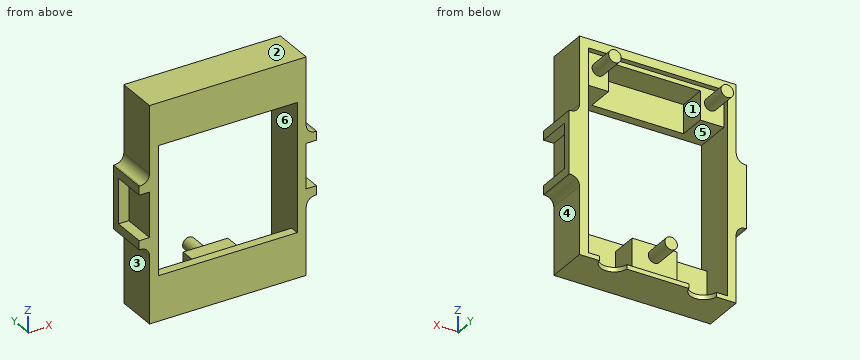
```python
from build123d import *

# Parameters (mm, degrees)
SKETCH1_W           = 35
SKETCH1_H           = 48
BOSS_EXTRUDE1_DEPTH = 2
SKETCH2_W           = 35
SKETCH2_H           = 48
SKETCH2_W_2         = 31
SKETCH2_H_2         = 44
BOSS_EXTRUDE2_DEPTH = 7.3
SKETCH3_W           = 10
SKETCH3_H           = 7
SKETCH3_W_2         = 5.25
SKETCH3_H_2         = 6.4
BOSS_EXTRUDE3_DEPTH = 6.1
CUT_EXTRUDE5_DEPTH  = 1
SKETCH10_W          = 31
SKETCH10_H          = 28.6
CUT_EXTRUDE6_DEPTH  = 31.586598372
BOSS_EXTRUDE4_START = 8.1
SKETCH8_R           = 1.4
BOSS_EXTRUDE4_DEPTH = 6
SKETCH14_W          = 2.3
SKETCH14_H          = 1.8
BOSS_EXTRUDE6_DEPTH = 5
SKETCH15_W          = 2
SKETCH15_H          = 9.3
BOSS_EXTRUDE7_DEPTH = 2.3
FILLET3_R           = 2
SKETCH16_W          = 31
SKETCH16_H          = 1
CUT_EXTRUDE8_DEPTH  = 1.2


with BuildPart() as part:
    # Sketch1 → Boss-Extrude1 (new body)
    with BuildSketch(Plane(origin=(0, 0, 0), x_dir=(1, 0, 0), z_dir=(0, 1, 0))):
        Rectangle(SKETCH1_W, SKETCH1_H)
    extrude(amount=BOSS_EXTRUDE1_DEPTH)

    # Sketch2 → Boss-Extrude2 (add)
    with BuildSketch(Plane(origin=(0, 2, 0), x_dir=(1, 0, 0), z_dir=(0, 1, 0))):
        Rectangle(SKETCH2_W, SKETCH2_H)
        with Locations((0, 1)):
            Rectangle(SKETCH2_W_2, SKETCH2_H_2, mode=Mode.SUBTRACT)
    extrude(amount=BOSS_EXTRUDE2_DEPTH)

    # Sketch3 → Boss-Extrude3 (add)
    with BuildSketch(Plane(origin=(0, 2, 0), x_dir=(1, 0, 0), z_dir=(0, 1, 0))):
        with Locations((0, 19.5)):
            Rectangle(SKETCH3_W, SKETCH3_H)
        with Locations((-12.875, -17.8)):
            Rectangle(SKETCH3_W_2, SKETCH3_H_2)
        with Locations((12.875, -17.8)):
            Rectangle(SKETCH3_W_2, SKETCH3_H_2)
    extrude(amount=BOSS_EXTRUDE3_DEPTH)

    # Sketch6 → Cut-Extrude5 (cut)
    with BuildSketch(Plane(origin=(0, 0, -24), x_dir=(-1, 0, 0), z_dir=(0, 0, -1))):
        with BuildLine():
            ThreePointArc((-13.059411708, 9.3), (-10, 6.7), (-6.940588292, 9.3))
            Line((-6.940588292, 9.3), (-13.059411708, 9.3))
        make_face()
        with BuildLine():
            Line((13.059411708, 9.3), (6.940588292, 9.3))
            ThreePointArc((6.940588292, 9.3), (10, 6.7), (13.059411708, 9.3))
        make_face()
    extrude(amount=-CUT_EXTRUDE5_DEPTH, mode=Mode.SUBTRACT)

    # Sketch10 → Cut-Extrude6 (cut, through all)
    with BuildSketch(Plane(origin=(0, 2, 0), x_dir=(1, 0, 0), z_dir=(0, 1, 0))):
        with Locations((0, -0.3)):
            Rectangle(SKETCH10_W, SKETCH10_H)
    extrude(amount=-CUT_EXTRUDE6_DEPTH, mode=Mode.SUBTRACT)

    # Sketch8 → Boss-Extrude4 (add)
    with BuildSketch(Plane(origin=(0, 0, 0), x_dir=(1, 0, 0), z_dir=(0, 1, 0)).offset(BOSS_EXTRUDE4_START)):
        with Locations(Location((-12.55, -18.7, 0), (0, 0, 90))):
            Circle(SKETCH8_R)
        with Locations(Location((12.55, -18.7, 0), (0, 0, 270))):
            Circle(SKETCH8_R)
        with Locations(Location((0, 18.6, 0), (0, 0, 270))):
            Circle(SKETCH8_R)
    extrude(amount=BOSS_EXTRUDE4_DEPTH)

    # Sketch14 → Boss-Extrude6 (add, symmetric)
    with BuildSketch(Plane.XY):
        with Locations((18.65, 8.4)):
            Rectangle(SKETCH14_W, SKETCH14_H)
    boss_extrude6 = extrude(amount=BOSS_EXTRUDE6_DEPTH, both=True)

    # Sketch15 → Boss-Extrude7 (add)
    with BuildSketch(Plane(origin=(17.5, 0, 0), x_dir=(0, 0, -1), z_dir=(1, 0, 0))):
        with Locations((-6, 4.65)):
            Rectangle(SKETCH15_W, SKETCH15_H)
        with Locations((6, 4.65)):
            Rectangle(SKETCH15_W, SKETCH15_H)
    boss_extrude7 = extrude(amount=BOSS_EXTRUDE7_DEPTH)

    # Mirror3: Boss-Extrude6, Boss-Extrude7 across plane
    add(boss_extrude6.mirror(Plane(origin=(0, 0, 0), x_dir=(0, 0, 1), z_dir=(1, 0, 0))))
    add(boss_extrude7.mirror(Plane(origin=(0, 0, 0), x_dir=(0, 0, 1), z_dir=(1, 0, 0))))

    # Fillet3
    fillet3_edges = [part.edges().sort_by_distance(p)[0] for p in [
        (17.5, 4.65, 7),
        (17.5, 4.65, -7),
        (-17.5, 4.65, 7),
        (-17.5, 4.65, -7),
    ]]
    fillet(fillet3_edges, radius=FILLET3_R)

    # Sketch16 → Cut-Extrude8 (cut)
    with BuildSketch(Plane(origin=(0, 9.3, 0), x_dir=(1, 0, 0), z_dir=(0, 1, 0))):
        with Locations((0, -21.5)):
            Rectangle(SKETCH16_W, SKETCH16_H)
    extrude(amount=-CUT_EXTRUDE8_DEPTH, mode=Mode.SUBTRACT)


solid = part.part
```
Work out the finished part from the listing and answer in its coordinate system (mm). Face numbers are marked on the shaded views. A direction names the side the tool comes from. Give positions to 0.01 mm unless a question says otherwise; leave off trailing zeros. Write each loop counter-clockwise with the first axis right and the second up, starting at its lowest first coordinate (ties: lowest second). Pieces come first, ordered by that corner, then holes. Notation, with made-up numbers: (16.5, -4.5) -> (45.5, -4.5) arc R29 cw to (45.5, 32.5) -> close; hole circle Ø8 at (49.25, 17.25). An arc over 180 degrees is marked (long way). Write item = value, one per line.
Q1. Section C-C on z = 16.5 is taken. Determine the outline of the cut face in (x, y), and give its area (3 significant figures).
Computed values:
outline = (-17.5, 0) -> (17.5, 0) -> (17.5, 9.3) -> (15.5, 9.3) -> (15.5, 8.1) -> (10.25, 8.1) -> (10.25, 2) -> (-10.25, 2) -> (-10.25, 8.1) -> (-15.5, 8.1) -> (-15.5, 9.3) -> (-17.5, 9.3) -> close
area = 163 mm^2
Q2. Flat-ended cylindrical pins translate along their axes: pin 1 Ø2.5 at (x, z) = (19, 0.5) entering from -Y; pin 2 Ø6 at (y, z) = (12, -14.5) entering from +X; pin 3 Ø1.8 at (x, y) = (19, 2.5) entering from +Z. Find the tip coordinate at first contact, or state that the pin passes through.
Computed values:
pin_1 = 7.5
pin_2 = 17.5
pin_3 = 7.57
Q3. Section A-A on z = -10.5 is taken. Determine the outline of the cut face in (x, y).
Computed values:
outline = (-17.5, 0) -> (-15.5, 0) -> (-15.5, 9.3) -> (-17.5, 9.3) -> close; (15.5, 0) -> (17.5, 0) -> (17.5, 9.3) -> (15.5, 9.3) -> close
Q4. Section D-D on x = 2.5 is taken. Determine the outline of the cut face in (y, z).
Computed values:
outline = (0, -24) -> (9.3, -24) -> (9.3, -23) -> (8.1, -23) -> (8.1, -16) -> (2, -16) -> (2, -14) -> (0, -14) -> close; (0, 14.6) -> (2, 14.6) -> (2, 21) -> (8.1, 21) -> (8.1, 22) -> (9.3, 22) -> (9.3, 24) -> (0, 24) -> close
Q5. For a pull along Z with two mould halves and no side action, classify the marked faces 1, 2 and 3 as pulls with the +Z half, pulls with the -Z half, needs draft (parallel to the pull), parting line crosses it, or undercut.
Computed values:
face_1 = undercut
face_2 = pulls with the +Z half
face_3 = needs draft
Q6. Consider line 1 along X through (y, z) = (6.75, -20); line 2 along Z through (x, y) = (6, 9); line 3 along X through (y, z) = (2.5, -1). Determine where each line is inside the solid, lowest interval first.
Computed values:
line_1 = -17.5 to -15.5, -5 to 5, 15.5 to 17.5
line_2 = -24 to -23, 22 to 24
line_3 = -17.5 to -15.5, 15.5 to 17.5
Q7. A tool of negligible diameter and unlimited length cuts with its end or side. For the marked faces 4, 5 and 6, from which of +Z, -Z, +X, -X, +Y, -Y can it reach the whole face along a straight path? Write none if from no direction.
Computed values:
face_4 = -Z, +X, +Y, -Y
face_5 = +Y, -Y
face_6 = +Y
Q8. Section B-B on x = 8 is taken. Determine the outline of the cut face in (y, z).
Computed values:
outline = (0, -24) -> (7.43, -24) -> (7.43, -23) -> (2, -23) -> (2, -14) -> (0, -14) -> close; (0, 14.6) -> (2, 14.6) -> (2, 21) -> (8.1, 21) -> (8.1, 22) -> (9.3, 22) -> (9.3, 24) -> (0, 24) -> close
